```python
from build123d import *

# Parameters (mm, degrees)
F0_W         = 203
F0_H         = 147
F1_DEPTH     = 45
F2_R         = 7
F3_DEPTH     = 3
F4_R         = 9
F5_DEPTH     = 10
F6_W         = 173
F6_H         = 34
F7_DEPTH     = 25
F8_T1_DEPTH  = 163
F8_T3_DEPTH  = 24
F8_T5_DEPTH  = 20
F8_S9_W      = 5
F8_S9_H      = 5
F8_T10_DEPTH = 5
F8_S15_W     = 5
F8_S15_H     = 5
F8_T16_DEPTH = 5
F8_S21_W     = 5
F8_S21_H     = 5
F8_T22_DEPTH = 5
F8_S27_W     = 5
F8_S27_H     = 5
F8_T28_DEPTH = 5
F8_T34_DEPTH = 22.5
F8_S36_R     = 9
F8_T37_DEPTH = 13
F8_T42_DEPTH = 10
F8_S43_R     = 9
F8_T44_DEPTH = 8
F8_T48_DEPTH = 10
F8_S49_R     = 9
F8_T50_DEPTH = 8
F9_W         = 18
F9_H         = 30
F10_DEPTH    = 10


# Not quite as in the source:
# - a fillet or chamfer that OpenCascade refuses, or shapes differently, is made with other operations: its cross-section is extruded or revolved along the edge and cut away or added


with BuildPart() as f1:
    # F0 (on Top) → F1 (new body)
    with BuildSketch(Plane.XY):
        with Locations((0, 73.5)):
            Rectangle(F0_W, F0_H)
    extrude(amount=F1_DEPTH)

    # F2 (on face) → F3 (join)
    with BuildSketch(Plane(origin=(0, 0, 0), x_dir=(1, 0, 0), z_dir=(0, 0, -1))):
        with Locations((-88.5, -14)):
            Circle(F2_R)
        with Locations((-88.5, -117)):
            Circle(F2_R)
        with Locations((88.5, -14)):
            Circle(F2_R)
        with Locations((88.5, -117)):
            Circle(F2_R)
    extrude(amount=F3_DEPTH)

    # F4 (on face) → F5 (join)
    with BuildSketch(Plane(origin=(0, 147, 0), x_dir=(-1, 0, 0), z_dir=(0, 1, 0))):
        with Locations((91, 8)):
            Circle(F4_R)
    extrude(amount=F5_DEPTH)

    # F6 (on face) → F7 (join)
    with BuildSketch(Plane(origin=(0, 147, 0), x_dir=(-1, 0, 0), z_dir=(0, 1, 0))):
        with Locations((0, 27)):
            Rectangle(F6_W, F6_H)
    extrude(amount=F7_DEPTH)

    # F8: fillet of radius 5 on 8 edges, made by hand

    # F8_s2 → F8_t1 (cut)
    with BuildSketch(Plane.YZ.offset(-81.5)):
        with BuildLine():
            ThreePointArc((172, 39), (170.5355339059, 42.5355339059), (167, 44))
            Line((167, 44), (172, 44))
            Line((172, 44), (172, 39))
        make_face()
        with BuildLine():
            ThreePointArc((167, 10), (170.5355339059, 11.4644660941), (172, 15))
            Line((172, 15), (172, 10))
            Line((172, 10), (167, 10))
        make_face()
    extrude(amount=F8_T1_DEPTH, mode=Mode.SUBTRACT)

    # F8_s4 → F8_t3 (cut)
    with BuildSketch(Plane.XY.offset(15)):
        with BuildLine():
            ThreePointArc((81.5, 172), (85.0355339059, 170.5355339059), (86.5, 167))
            Line((86.5, 167), (86.5, 172))
            Line((86.5, 172), (81.5, 172))
        make_face()
        with BuildLine():
            ThreePointArc((-81.5, 172), (-85.0355339059, 170.5355339059), (-86.5, 167))
            Line((-86.5, 167), (-86.5, 172))
            Line((-86.5, 172), (-81.5, 172))
        make_face()
    extrude(amount=F8_T3_DEPTH, mode=Mode.SUBTRACT)

    # F8_s6 → F8_t5 (cut)
    with BuildSketch(Plane.XZ.offset(-167)):
        with BuildLine():
            ThreePointArc((86.5, 39), (85.0355339059, 42.5355339059), (81.5, 44))
            Line((81.5, 44), (86.5, 44))
            Line((86.5, 44), (86.5, 39))
        make_face()
        with BuildLine():
            ThreePointArc((81.5, 10), (85.0355339059, 11.4644660941), (86.5, 15))
            Line((86.5, 15), (86.5, 10))
            Line((86.5, 10), (81.5, 10))
        make_face()
        with BuildLine():
            ThreePointArc((-81.5, 44), (-85.0355339059, 42.5355339059), (-86.5, 39))
            Line((-86.5, 39), (-86.5, 44))
            Line((-86.5, 44), (-81.5, 44))
        make_face()
    extrude(amount=F8_T5_DEPTH, mode=Mode.SUBTRACT)


with BuildPart() as f8_tool8:
    # F8_s9 → F8_t10 (new body)
    with BuildSketch(Plane.XZ.offset(-167)):
        with Locations((-84, 41.5)):
            Rectangle(F8_S9_W, F8_S9_H)
    extrude(amount=-F8_T10_DEPTH)

    # F8_s11 → F8_t12 (revolve, cut)
    with BuildSketch(Plane(origin=(-81.5, 167, 39), x_dir=(0.7071067812, 0, -0.7071067812), z_dir=(0.7071067812, 0, 0.7071067812))):
        with BuildLine():
            ThreePointArc((0, -5), (5, 0), (0, 5))
            Line((0, 5), (0, -5))
        make_face()
    revolve(axis=Axis((-81.5, 167, 39), (0, 1, 0)), mode=Mode.SUBTRACT)


with BuildPart() as f1_1:
    add(f1.part)

    # F8_t7: cut F8_tool8
    add(f8_tool8.part, mode=Mode.SUBTRACT)


with BuildPart() as f8_tool14:
    # F8_s15 → F8_t16 (new body)
    with BuildSketch(Plane.XZ.offset(-167)):
        with Locations((84, 41.5)):
            Rectangle(F8_S15_W, F8_S15_H)
    extrude(amount=-F8_T16_DEPTH)

    # F8_s17 → F8_t18 (revolve, cut)
    with BuildSketch(Plane(origin=(81.5, 167, 39), x_dir=(-0.7071067812, 0, -0.7071067812), z_dir=(0.7071067812, 0, -0.7071067812))):
        with BuildLine():
            ThreePointArc((0, -5), (5, 0), (0, 5))
            Line((0, 5), (0, -5))
        make_face()
    revolve(axis=Axis((81.5, 167, 39), (0, 1, 0)), mode=Mode.SUBTRACT)


with BuildPart() as f1_2:
    add(f1_1.part)

    # F8_t13: cut F8_tool14
    add(f8_tool14.part, mode=Mode.SUBTRACT)


with BuildPart() as f8_tool20:
    # F8_s21 → F8_t22 (new body)
    with BuildSketch(Plane.XY.offset(15)):
        with Locations((84, 169.5)):
            Rectangle(F8_S21_W, F8_S21_H)
    extrude(amount=-F8_T22_DEPTH)

    # F8_s23 → F8_t24 (revolve, cut)
    with BuildSketch(Plane(origin=(81.5, 167, 15), x_dir=(-0.7071067812, -0.7071067812, 0), z_dir=(0.7071067812, -0.7071067812, 0))):
        with BuildLine():
            ThreePointArc((0, -5), (5, 0), (0, 5))
            Line((0, 5), (0, -5))
        make_face()
    revolve(axis=Axis((81.5, 167, 15), (0, 0, -1)), mode=Mode.SUBTRACT)


with BuildPart() as f1_3:
    add(f1_2.part)

    # F8_t19: cut F8_tool20
    add(f8_tool20.part, mode=Mode.SUBTRACT)


with BuildPart() as f8_tool26:
    # F8_s27 → F8_t28 (new body)
    with BuildSketch(Plane.XY.offset(15)):
        with Locations((-84, 169.5)):
            Rectangle(F8_S27_W, F8_S27_H)
    extrude(amount=-F8_T28_DEPTH)

    # F8_s29 → F8_t30 (revolve, cut)
    with BuildSketch(Plane(origin=(-81.5, 167, 15), x_dir=(0.7071067812, -0.7071067812, 0), z_dir=(0.7071067812, 0.7071067812, 0))):
        with BuildLine():
            ThreePointArc((0, -5), (5, 0), (0, 5))
            Line((0, 5), (0, -5))
        make_face()
    revolve(axis=Axis((-81.5, 167, 15), (0, 0, -1)), mode=Mode.SUBTRACT)


with BuildPart() as f1_4:
    add(f1_3.part)

    # F8_t25: cut F8_tool26
    add(f8_tool26.part, mode=Mode.SUBTRACT)


with BuildPart() as f8_tool32:
    # F8_s33 → F8_t34 (new body)
    with BuildSketch(Plane.XZ.offset(-144.5)):
        with BuildLine():
            ThreePointArc((-81.5, 10), (-85.0355339059, 11.4644660941), (-86.5, 15))
            Line((-86.5, 15), (-86.5, 10))
            Line((-86.5, 10), (-81.5, 10))
        make_face()
    extrude(amount=-F8_T34_DEPTH)

    split(bisect_by=Plane.XZ.offset(-147), keep=Keep.BOTTOM)

    # F8_s36 → F8_t37 (cut, symmetric)
    with BuildSketch(Plane.XZ.offset(-155.8)):
        with Locations((-91, 8)):
            Circle(F8_S36_R)
    extrude(amount=F8_T37_DEPTH, both=True, mode=Mode.SUBTRACT)

    split(bisect_by=Plane.XZ.offset(-157), keep=Keep.TOP)


with BuildPart() as f1_5:
    add(f1_4.part)

    # F8_t31: cut F8_tool32
    add(f8_tool32.part, mode=Mode.SUBTRACT)


with BuildPart() as f8_tool40:
    # F8_s41 → F8_t42 (new body)
    with BuildSketch(Plane.XZ.offset(-157)):
        with BuildLine():
            ThreePointArc((-81.5, 10), (-85.0355339059, 11.4644660941), (-86.5, 15))
            Line((-86.5, 15), (-86.5, 10))
            Line((-86.5, 10), (-81.5, 10))
        make_face()
    extrude(amount=-F8_T42_DEPTH)

    # F8_s43 → F8_t44 (cut, symmetric)
    with BuildSketch(Plane.XZ.offset(-162)):
        with Locations((-91, 8)):
            Circle(F8_S43_R)
    extrude(amount=F8_T44_DEPTH, both=True, mode=Mode.SUBTRACT)


with BuildPart() as f1_6:
    add(f1_5.part)

    # F8_t39: cut F8_tool40
    add(f8_tool40.part, mode=Mode.SUBTRACT)


with BuildPart() as f8_tool46:
    # F8_s47 → F8_t48 (new body)
    with BuildSketch(Plane.XZ.offset(-157)):
        with BuildLine():
            ThreePointArc((-81.5, 10), (-85.0355339059, 11.4644660941), (-86.5, 15))
            Line((-86.5, 15), (-86.5, 10))
            Line((-86.5, 10), (-81.5, 10))
        make_face()
    extrude(amount=-F8_T48_DEPTH)

    # F8_s49 → F8_t50 (intersect, symmetric)
    with BuildSketch(Plane.XZ.offset(-162)):
        with Locations((-91, 8)):
            Circle(F8_S49_R)
    extrude(amount=F8_T50_DEPTH, both=True, mode=Mode.INTERSECT)


with BuildPart() as f1_7:
    add(f1_6.part)

    # F8_t45: cut F8_tool46
    add(f8_tool46.part, mode=Mode.SUBTRACT)

    # F9 (on face) → F10 (join, through all)
    with BuildSketch(Plane(origin=(0, 157, 0), x_dir=(-1, 0, 0), z_dir=(0, 1, 0))):
        with Locations((91, 23)):
            Rectangle(F9_W, F9_H)
    extrude(amount=-F10_DEPTH)


solid = f1_7.part
```
Work out the finished part from the listing and answer in its coordinate system (mm). A direction names the side the tool comes from. Give positions to 0.01 mm unless a question says otherwise; leave off trailing zeros. Loops run counter-clockwise (first coordinate to the right, second up) from the corner with the lowest first, then second, coordinate; pieces in that order, holes last. Notation, with made-up numbers: (8.5, -34.75) -> (26.5, -34.75) arc R14 ccw to (26.5, -16.75) -> close; hole circle Ø11 at (75, -11.5). An arc over 180 degrees is marked (long way). Use CSV: the item, a comma, the result in double quotes.
1. The part is cut by section D-D (z = 3). Write down the section's boundary in (x, y), then the cut area to 3 significant figures.
Found:
outline,"(-101.5, 0) -> (101.5, 0) -> (101.5, 147) -> (-83.52, 147) -> (-83.52, 157) -> (-98.48, 157) -> (-98.48, 147) -> (-101.5, 147) -> close"
area,"30,000 mm^2"
2. The part is cut by section C-C (y = 14). Write down the section's boundary in (x, z).
Found:
outline,"(-101.5, 0) -> (-95.5, 0) -> (-95.5, -3) -> (-81.5, -3) -> (-81.5, 0) -> (81.5, 0) -> (81.5, -3) -> (95.5, -3) -> (95.5, 0) -> (101.5, 0) -> (101.5, 45) -> (-101.5, 45) -> close"
3. The mould has two halves that part along Y. Classify faces 4 (the cylindrical face through (82.945, 121.259, -1.479)), 5 (the flat face through (-93, 152, 38)), 6 (the cylindrical face through (-85, 170.57, 26.83)), 7 (the cylindrical face through (81.507, 13.692, -1.479)): +Y half, -Y half, draft (parallel to the pull), parting line (faces both ways), or undercut.
Found:
face 4,"undercut"
face 5,"draft"
face 6,"+Y half"
face 7,"undercut"
4. The part is cut by section B-B (z = 27.5). Write down the section's boundary in (x, y).
Found:
outline,"(-101.5, 0) -> (101.5, 0) -> (101.5, 147) -> (86.5, 147) -> (86.5, 167) arc R5 ccw to (81.5, 172) -> (-81.5, 172) arc R5 ccw to (-86.5, 167) -> (-86.5, 157) -> (-100, 157) -> (-100, 147) -> (-101.5, 147) -> close"
5. A tool of negligible diameter and unlimited length cuts with its end or side. For faces 1 (the flat face through (1, 157, 44)), 2 (the flat face through (-1, 75, 0)), 3 (the flat face through (1, 172, 27)), from which of +Z, -Z, +X, -X, +Y, -Y can it reach the whole face along a straight path? Write none if from no direction.
Found:
face 1,"+Z, +X, -X, +Y"
face 2,"-Z"
face 3,"+Z, -Z, +X, -X, +Y"
6. Flat-ended cylindrical pins translate along their axes: pin 1 Ø14.5 at (x, z) = (-95, 24.5) entering from +Y; pin 2 Ø3 at (y, z) = (152, 28.5) entering from -X; pin 3 Ø1 at (x, y) = (-39.5, 153) entering from +Z; pin 4 Ø8 at (x, z) = (23, 15) entering from -Y. Find the tip coordinate at first contact, or state that the pin passes through.
Found:
pin 1,"y = 157"
pin 2,"x = -100"
pin 3,"z = 44"
pin 4,"y = 0"
7. Straight lines are drawn through the part: line 1 (Z direction, x = -76.5, y = 151.5); line 2 (Z direction, x = 63, y = 36.5); line 3 (X direction, y = 160.5, z = 21). For each, find the intervals that lie inside material, in ascending order.
Found:
line 1,"10 to 44"
line 2,"0 to 45"
line 3,"-86.5 to 86.5"
8. The part is cut by section A-A (x = -25). Write down the section's boundary in (y, z).
Found:
outline,"(0, 0) -> (147, 0) -> (147, 10) -> (167, 10) arc R5 ccw to (172, 15) -> (172, 39) arc R5 ccw to (167, 44) -> (147, 44) -> (147, 45) -> (0, 45) -> close"
